from build123d import *

# Parameters (mm, degrees)
SKETCH_1_R               = 28.5
EXTRUDE_1_DEPTH          = 52.25
SKETCH_2_R               = 1.5
CUT_EXTRUDE_1_DEPTH      = 5
PATTERN_CIRCULAR_1_COUNT = 6
SKETCH_3_R               = 17.5
CUT_EXTRUDE_2_DEPTH      = 10
CUT_EXTRUDE_START        = -1
CUT_EXTRUDE_5_DEPTH      = 5
CUT_EXTRUDE_6_DEPTH      = 8
SKETCH_8_R               = 1.5
CUT_EXTRUDE_8_DEPTH      = 4
PATTERN_CIRCULAR_2_COUNT = 4


with BuildPart() as part:
    # 草图1 → 凸台-拉伸1 (new body)
    with BuildSketch(Plane.XY):
        Circle(SKETCH_1_R)
    extrude(amount=EXTRUDE_1_DEPTH)

    # 草图2 → 切除-拉伸1 (cut)
    with BuildSketch(Plane.XY.offset(52.25)):
        with Locations((25, 0)):
            Circle(SKETCH_2_R)
    cut_extrude_1 = extrude(amount=-CUT_EXTRUDE_1_DEPTH, mode=Mode.SUBTRACT)

    # 阵列(圆周)1: 切除-拉伸1 ×6 about axis
    pattern_circular_1_axis = Axis((0, 0, 0), (0, 0, 1))
    for i in range(1, PATTERN_CIRCULAR_1_COUNT):
        add(cut_extrude_1.rotate(pattern_circular_1_axis, i * 360 / PATTERN_CIRCULAR_1_COUNT), mode=Mode.SUBTRACT)

    # 草图3 → 切除-拉伸2 (cut)
    with BuildSketch(Plane.XY.offset(52.25)):
        Circle(SKETCH_3_R)
    extrude(amount=-CUT_EXTRUDE_2_DEPTH, mode=Mode.SUBTRACT)

    # 草图5 → 切除-拉伸5 (cut)
    with BuildSketch(Plane(origin=(0, 0, 0), x_dir=(-1, 0, 0), z_dir=(0, 0, -1)).offset(CUT_EXTRUDE_START)):
        with BuildLine():
            ThreePointArc((28.5, 0), (28.280902723, 3.527115134), (27.626979567, 7))
            Line((27.626979567, 7), (25.5, 7))
            Line((25.5, 7), (25.5, -7))
            Line((25.5, -7), (27.626979567, -7))
            ThreePointArc((27.626979567, -7), (28.280902723, -3.527115134), (28.5, 0))
        make_face()
        with BuildLine():
            Line((-25.5, 7), (-27.626979567, 7))
            ThreePointArc((-27.626979567, 7), (-28.5, 0), (-27.626979567, -7))
            Line((-27.626979567, -7), (-25.5, -7))
            Line((-25.5, -7), (-25.5, 7))
        make_face()
    extrude(amount=-CUT_EXTRUDE_5_DEPTH, mode=Mode.SUBTRACT)

    # 草图7 → 切除-拉伸6 (cut)
    with BuildSketch(Plane(origin=(0, 0, 0), x_dir=(-1, 0, 0), z_dir=(0, 0, -1)).offset(CUT_EXTRUDE_START)):
        with BuildLine():
            Line((-4, -28.217902119), (-4, -25.5))
            Line((-4, -25.5), (4, -25.5))
            Line((4, -25.5), (4, -28.217902119))
            ThreePointArc((4, -28.217902119), (0, -28.5), (-4, -28.217902119))
        make_face()
    extrude(amount=-CUT_EXTRUDE_6_DEPTH, mode=Mode.SUBTRACT)

    # 草图8 → 切除-拉伸8 (cut)
    with BuildSketch(Plane(origin=(0, 0, 0), x_dir=(-1, 0, 0), z_dir=(0, 0, -1))):
        with Locations((13.435028843, 13.435028843)):
            Circle(SKETCH_8_R)
    cut_extrude_8 = extrude(amount=-CUT_EXTRUDE_8_DEPTH, mode=Mode.SUBTRACT)

    # 阵列(圆周)2: 切除-拉伸8 ×4 about axis
    pattern_circular_2_axis = Axis((0, 0, 0), (0, 0, 1))
    for i in range(1, PATTERN_CIRCULAR_2_COUNT):
        add(cut_extrude_8.rotate(pattern_circular_2_axis, i * 360 / PATTERN_CIRCULAR_2_COUNT), mode=Mode.SUBTRACT)


solid = part.part
Geometry: final body of the model. Coordinates: model frame, mm. A direction names the side the tool comes from. Give positions to 0.01 mm unless a question says otherwise; leave off trailing zeros. Write each loop counter-clockwise with the first axis right and the second up, starting at its lowest first coordinate (ties: lowest second). Pieces come first, ordered by that corner, then holes. Notation, with made-up numbers: (32.25, -38) -> (41.25, -38) arc R23 cw to (41.25, -28) -> close; hole circle Ø4 at (39, 39.5). An arc over 180 degrees is marked (long way). Answer in a Markdown table with one row per item.
(1) Set-up query: faces 1 (the flat face through (27, -7, 3)), 2 (the flat face through (13, -13, 4)), 3 (the cylindrical face through (-11.694, 22.915, 49.785)), 4 (the flat face through (0, -27, 1)). Return all of +Z, -Z, +X, -X, +Y, -Y with unobstructed straight access to the full face (end or side cutting, diameter ignored); none if empty.
Answers below:
| item | result |
|---|---|
| face 1 | +X |
| face 2 | -Z |
| face 3 | +Z |
| face 4 | -Y |
(2) Section query C-C on x = -2.5. Return loops of the section in (y, z).
Answers below:
| item | result |
|---|---|
| outline | (-28.39, 0) -> (28.39, 0) -> (28.39, 52.25) -> (17.32, 52.25) -> (17.32, 42.25) -> (-17.32, 42.25) -> (-17.32, 52.25) -> (-28.39, 52.25) -> (-28.39, 9) -> (-25.5, 9) -> (-25.5, 1) -> (-28.39, 1) -> close |
(3) Pin query (flat end, axial travel): pin 1 (5 mm diameter, centred on x = 13.44, y = 13.44, fed in from -Z); pin 2 (10 mm diameter, centred on x = -22, z = 14.5, fed in from +Y); pin 3 (4 mm diameter, centred on y = -9.5, z = 31, fed in from -X); pin 4 (1.5 mm diameter, centred on x = 24.5, y = 0, fed in from +Z). Return the tip coordinate at first contact, or that it passes through.
Answers below:
| item | result |
|---|---|
| pin 1 | z = 0 |
| pin 2 | y = 22.87 |
| pin 3 | x = -27.5 |
| pin 4 | z = 47.25 |
(4) Ray query, line 1 along Y through (x, z) = (12, 50); line 2 along Z through (x, y) = (4, -15); line 3 along Y through (x, z) = (-25, 50.75). Return the intervals inside material, ascending. Write a range as [from, to].
Answers below:
| item | result |
|---|---|
| line 1 | [-25.85, -23.06], [-20.24, -12.74], [12.74, 20.24], [23.06, 25.85] |
| line 2 | [0, 42.25] |
| line 3 | [-13.68, -1.5], [1.5, 13.68] |
(5) Section query A-A on y = 0. Return loops of the section in (x, z), then the cut area to 3 significant figures.
Answers below:
| item | result |
|---|---|
| outline | (-28.5, 0) -> (28.5, 0) -> (28.5, 1) -> (25.5, 1) -> (25.5, 6) -> (28.5, 6) -> (28.5, 52.25) -> (26.5, 52.25) -> (26.5, 47.25) -> (23.5, 47.25) -> (23.5, 52.25) -> (17.5, 52.25) -> (17.5, 42.25) -> (-17.5, 42.25) -> (-17.5, 52.25) -> (-23.5, 52.25) -> (-23.5, 47.25) -> (-26.5, 47.25) -> (-26.5, 52.25) -> (-28.5, 52.25) -> (-28.5, 6) -> (-25.5, 6) -> (-25.5, 1) -> (-28.5, 1) -> close |
| area | 2,570 mm^2 |
(6) Section query D-D on y = -11. Return loops of the section in (x, z).
Answers below:
| item | result |
|---|---|
| outline | (-26.29, 0) -> (26.29, 0) -> (26.29, 52.25) -> (13.61, 52.25) -> (13.61, 42.25) -> (-13.61, 42.25) -> (-13.61, 52.25) -> (-26.29, 52.25) -> close |
(7) Section query B-B on z = 30.5. Return loops of the section in (x, y), then the cut area to 3 significant figures.
Answers below:
| item | result |
|---|---|
| outline | circle Ø57 at (0, 0) |
| area | 2,550 mm^2 |
(8) Draft query along X for faces 5 (the cylindrical face through (-23.5, -0.07, 49.78)), 6 (the flat face through (-27, 7, 3)). Return one class per face: +X half, -X half, draft (parallel to the pull), parting line (faces both ways), or undercut.
Answers below:
| item | result |
|---|---|
| face 5 | undercut |
| face 6 | draft |
